from build123d import *

# Parameters (mm, degrees)
BOSS_EXTRUDE1_DEPTH = 3
SKETCH3_R           = 2
CUT_EXTRUDE1_DEPTH  = 46.565886362


with BuildPart() as part:
    # Sketch1 → Boss-Extrude1 (new body)
    with BuildSketch(Plane(origin=(0, 0, 0), x_dir=(1, 0, 0), z_dir=(0, 1, 0))):
        with BuildLine():
            Line((-44, -6.5), (44, -6.5))
            ThreePointArc((44, -6.5), (44.707106781, -6.207106781), (45, -5.5))
            Line((45, -5.5), (45, 5.5))
            ThreePointArc((45, 5.5), (44.707106781, 6.207106781), (44, 6.5))
            Line((44, 6.5), (-44, 6.5))
            ThreePointArc((-44, 6.5), (-44.707106781, 6.207106781), (-45, 5.5))
            Line((-45, 5.5), (-45, -5.5))
            ThreePointArc((-45, -5.5), (-44.707106781, -6.207106781), (-44, -6.5))
        make_face()
    extrude(amount=BOSS_EXTRUDE1_DEPTH)

    # Sketch3 → Cut-Extrude1 (cut, through all)
    with BuildSketch(Plane(origin=(0, 3, 0), x_dir=(1, 0, 0), z_dir=(0, 1, 0))):
        with Locations(Location((-40, 0, 0), (0, 0, 270))):
            Circle(SKETCH3_R)
        with Locations(Location((-28.571428571, 0, 0), (0, 0, 270))):
            Circle(SKETCH3_R)
        with Locations(Location((-17.142857143, 0, 0), (0, 0, 270))):
            Circle(SKETCH3_R)
        with Locations(Location((-5.714285714, 0, 0), (0, 0, 270))):
            Circle(SKETCH3_R)
        with Locations(Location((5.714285714, 0, 0), (0, 0, 270))):
            Circle(SKETCH3_R)
        with Locations(Location((17.142857143, 0, 0), (0, 0, 270))):
            Circle(SKETCH3_R)
        with Locations(Location((28.571428571, 0, 0), (0, 0, 270))):
            Circle(SKETCH3_R)
        with Locations(Location((40, 0, 0), (0, 0, 270))):
            Circle(SKETCH3_R)
    extrude(amount=-CUT_EXTRUDE1_DEPTH, mode=Mode.SUBTRACT)


solid = part.part
Part model, mm, in its own coordinate system. Coordinates: 2 decimals unless noted, no trailing zeros. Order: outer loops, then holes, each group sorted by start corner. A loop starts at its lowest first (then second) coordinate and runs counter-clockwise, first axis right, second up. Notation, with made-up numbers: M -22.75,-37.5 L 7.25,-37.5 A18 cw 7.25,-14.5 Z; hole C 26,46.5 d1. An arc over 180 degrees is marked long. One line per question, with ' | ' between items.
Q1. Drill centre lines: line 1 (Z direction, x = -15.5, y = 1.05); line 2 (Z direction, x = -17.5, y = 0.4); line 3 (X direction, y = 2.75, z = -5.75). Where is each one in solid material? Low to high.
A:
line 1: z = -6.5 to -1.14, 1.14 to 6.5 | line 2: z = -6.5 to -1.97, 1.97 to 6.5 | line 3: x = -44.97 to 44.97
Q2. Slice it at A-A (x = -40). Give the cut face in (y, z), and give its area (3 significant figures).
A:
outline: M 0,-6.5 L 3,-6.5 L 3,-2 L 0,-2 Z; M 0,2 L 3,2 L 3,6.5 L 0,6.5 Z | area: 27.0 mm^2
Q3. Two-plate mould, pull along X, no slides. Class faces 1 (the face through (-42, 2, 0)), 2 (the face through (-1, 0, 0)), 3 (the face through (-45, 1, 0)): +X half, -X half, draft (parallel to the pull), parting line (faces both ways), or undercut.
A:
face 1: undercut | face 2: draft | face 3: -X half
Q4. Slice it at B-B (y = 1.4). Count the separate pieces of the cut face and the enclosed holes in it, and give its area (3 significant figures).
A:
separate pieces: 1 | enclosed holes: 8 | area: 1,070 mm^2
